Here's how the part is built. I have some questions about the finished solid (model axes, mm). A direction names the side the tool comes from. Coordinates: 2 decimals unless noted, no trailing zeros. Loops run counter-clockwise (first coordinate to the right, second up) from the corner with the lowest first, then second, coordinate; pieces in that order, holes last. Notation, with made-up numbers: (49, 1.5) -> (92, 1.5) arc R17 ccw to (92, 14.5) -> close; hole circle Ø7 at (81.25, 0.5). An arc over 180 degrees is marked (long way). Use CSV: the item, a comma, the result in double quotes. Start each with the question number.
from build123d import *

# Parameters (mm, degrees)
SKETCH_1_W                   = 270
SKETCH_1_H                   = 180
EXTRUDE_1_DEPTH              = 15
CHAMFER_1_SIZE               = 5
HOLE_WIZARD_M8_1_D           = 8.4
HOLE_WIZARD_M8_1_CBORE_D     = 15
HOLE_WIZARD_M8_1_CBORE_DEPTH = 8
CUT_EXTRUDE_1_DEPTH          = 325.846117416


with BuildPart() as part:
    # 草图1 → 凸台-拉伸1 (new body)
    with BuildSketch(Plane.XY):
        with Locations((135, 90)):
            Rectangle(SKETCH_1_W, SKETCH_1_H)
    extrude(amount=EXTRUDE_1_DEPTH)

    # 倒角1
    chamfer_1_edges = [part.edges().sort_by_distance(p)[0] for p in [
        (0, 180, 7.5),
        (270, 180, 7.5),
        (270, 0, 7.5),
        (0, 0, 7.5),
    ]]
    chamfer(chamfer_1_edges, length=CHAMFER_1_SIZE)

    # M8 凹头盖螺钉的柱形沉头孔1 (through all)
    with Locations(Plane(origin=(0, 0, 0), x_dir=(-1, 0, 0), z_dir=(0, 0, -1))):
        with Locations((-240, 90), (-30, 90), (-135, 30), (-135, 150)):
            CounterBoreHole(HOLE_WIZARD_M8_1_D / 2, HOLE_WIZARD_M8_1_CBORE_D / 2, HOLE_WIZARD_M8_1_CBORE_DEPTH)

    # 草图4 → 切除-拉伸1 (cut, through all)
    with BuildSketch(Plane(origin=(0, 180, 0), x_dir=(1, 0, 0), z_dir=(0, 1, 0))):
        Polygon((55, -9), (71, -9), (71, -3), (67.5, -3), (67.5, 0), (58.5, 0), (58.5, -3), (55, -3), align=None)
        Polygon((202.5, -3), (199, -3), (199, -9), (215, -9), (215, -3), (211.5, -3), (211.5, 0), (202.5, 0), align=None)
    extrude(amount=-CUT_EXTRUDE_1_DEPTH, mode=Mode.SUBTRACT)


solid = part.part
1) I want a section at B-B, the plane x = 30. Please give me the cut outline in (y, z), plus the area to 3 significant figures.
2) Please list where these lines run through material, in increasing order: L1, parallel to Y at x = 135, z = 13; L2, parallel to X at y = 18, z = 5.25; L3, parallel to Y at x = 240, z = 5.5. Write a range as [from, to].
3) For P1, Ø6.5, axis at x = 240, y = 90, coming from the +Z side; P2, Ø4.5, axis at x = 242.5, y = 92, coming from the -Z side; P3, Ø5, axis at x = 64, y = 105.5, coming from the -Z side, each with a flat end and sliding along its axis, tell me the tip position at first contact or that it passes through.
4) I want a section at A-A, the plane y = 30. Please give me the cut outline in (x, z), plus the area to 3 significant figures.
5) Thinking about a two-plate mould opening in X: for faces 4 (the face through (133, 0, 7)), 5 (the face through (0, 89, 7)), 6 (the face through (71, 91, 6)), which applies, pulls with the +X half, pulls with the -X half, needs draft (parallel to the pull), parting line crosses it, or undercut?
6) I want a section at D-D, the plane x = 206. Please give me the cut outline in (y, z), plus the area to 3 significant figures.
7) I want a section at C-C, the plane y = 90. State how many separate pieces and enclosed holes the cut face has, plus the area to 3 significant figures.
8) Which directions (+Z, -Z, +X, -X, +Y, -Y) give clear straight access to the entire face, cutting with the end or side of a thin tool? Please do faces 1 (the face through (55, 91, 6)), 2 (the face through (243.88, 88.39, 11.55)), 3 (the face through (241.63, 82.68, 3.94)).
Return value:
1,outline,"(0, 0) -> (82.5, 0) -> (82.5, 8) -> (85.8, 8) -> (85.8, 15) -> (0, 15) -> close; (94.2, 8) -> (97.5, 8) -> (97.5, 0) -> (180, 0) -> (180, 15) -> (94.2, 15) -> close"
1,area,"2,520 mm²"
2,L1,"y = [0, 25.8], [34.2, 145.8], [154.2, 180]"
2,L2,"x = [0, 55], [71, 199], [215, 270]"
2,L3,"y = [0, 82.5], [97.5, 180]"
3,P1,"passes through"
3,P2,"stops at z = 8"
3,P3,"stops at z = 9"
4,outline,"(0, 0) -> (58.5, 0) -> (58.5, 3) -> (55, 3) -> (55, 9) -> (71, 9) -> (71, 3) -> (67.5, 3) -> (67.5, 0) -> (127.5, 0) -> (127.5, 8) -> (130.8, 8) -> (130.8, 15) -> (0, 15) -> close; (139.2, 8) -> (142.5, 8) -> (142.5, 0) -> (202.5, 0) -> (202.5, 3) -> (199, 3) -> (199, 9) -> (215, 9) -> (215, 3) -> (211.5, 3) -> (211.5, 0) -> (270, 0) -> (270, 15) -> (139.2, 15) -> close"
4,area,"3,630 mm²"
5,face 4,"needs draft"
5,face 5,"pulls with the -X half"
5,face 6,"undercut"
6,outline,"(0, 9) -> (180, 9) -> (180, 15) -> (0, 15) -> close"
6,area,"1,080 mm²"
7,separate pieces,"3"
7,enclosed holes,"0"
7,area,"3,450 mm²"
8,face 1,"+Y, -Y"
8,face 2,"+Z, -Z"
8,face 3,"-Z"
